Read the model definition and answer for the solid it produces. Units are mm, in the model's axes. A direction names the side the tool comes from. Give positions to 0.01 mm unless a question says otherwise; leave off trailing zeros. Write each loop counter-clockwise with the first axis right and the second up, starting at its lowest first coordinate (ties: lowest second). Pieces come first, ordered by that corner, then holes. Notation, with made-up numbers: M 13.25,79.5 L 61.25,79.5 A23 cw 61.25,94.5 Z; hole C 77.5,25 d3. An arc over 180 degrees is marked long. Put each result on its own line as item: value.
Autodesk Inventor part; units mm, degrees
ref_plane "YZ Plane" through (0, 0, 0) normal (1, 0, 0) x (0, 1, 0)
ref_plane "XZ Plane" through (0, 0, 0) normal (0, 1, 0) x (-1, 0, 0)
ref_plane "XY Plane" through (0, 0, 0) normal (0, 0, 1) x (1, 0, 0)
sketch "Sketch1" plane through (0, 0, 0) normal (0, 1, 0) x (-1, 0, 0)
  line L0 (0, 69.85) -> (0, -69.85)
  line L1 (2.54, 69.85) -> (10.16, 69.85)
  line L2 (10.16, 67.31) -> (10.16, 64.77)
  line L3 (10.16, 64.77) -> (7.9419, 64.217)
  line L4 (10.16, 58.674) -> (7.9419, 59.227)
  arc A0 (7.9419, 64.217) -> (7.9419, 59.227) centre (5.9783, 61.722) ccw
  line L5 (0, 69.85) -> (2.54, 69.85)
  line L6 (6.604, 69.85) -> (2.794, 69.85)
  line L7 (2.794, 69.85) -> (2.794, 82.55)
  line L8 (2.794, 82.55) -> (6.604, 82.55)
  line L9 (6.604, 82.55) -> (6.604, 69.85)
  line L10 (2.54, -69.85) -> (2.54, -81.28)
  line L11 (2.54, -81.28) -> (0, -81.28)
  line L12 (0, -81.28) -> (0, -69.85)
  line L13 (5.9783, 61.722) -> (7.9419, 61.722) construction
  line L14 (7.9419, 61.722) -> (7.9419, 59.227) construction
  line L15 (7.9419, 61.722) -> (7.9419, 64.217) construction
  line L16 (10.16, 67.31) -> (10.16, 69.85)
  line L17 (10.16, -66.802) -> (10.16, -69.85)
  line L18 (10.16, -69.85) -> (2.54, -69.85)
  line L19 (10.16, 58.674) -> (10.16, 56.134)
  line L20 (10.16, 56.134) -> (10.16, 53.594)
  line L21 (10.16, 53.594) -> (7.9419, 53.041)
  line L22 (7.9419, 50.546) -> (7.9419, 53.041) construction
  arc A1 (7.9419, 53.041) -> (7.9419, 48.051) centre (5.9783, 50.546) ccw
  line L23 (7.9419, 50.546) -> (7.9419, 48.051) construction
  line L24 (10.16, 47.498) -> (7.9419, 48.051)
  line L25 (10.16, 47.498) -> (10.16, 44.958)
  line L26 (5.9783, 50.546) -> (7.9419, 50.546) construction
  line L27 (10.16, 44.958) -> (10.16, 42.418)
  line L28 (10.16, 42.418) -> (7.9419, 41.865)
  line L29 (7.9419, 39.37) -> (7.9419, 41.865) construction
  arc A2 (7.9419, 41.865) -> (7.9419, 36.875) centre (5.9783, 39.37) ccw
  line L30 (7.9419, 39.37) -> (7.9419, 36.875) construction
  line L31 (10.16, 36.322) -> (7.9419, 36.875)
  line L32 (10.16, 36.322) -> (10.16, 33.782)
  line L33 (5.9783, 39.37) -> (7.9419, 39.37) construction
  line L34 (10.16, 33.782) -> (10.16, 31.242)
  line L35 (10.16, 31.242) -> (7.9419, 30.689)
  line L36 (7.9419, 28.194) -> (7.9419, 30.689) construction
  arc A3 (7.9419, 30.689) -> (7.9419, 25.699) centre (5.9783, 28.194) ccw
  line L37 (7.9419, 28.194) -> (7.9419, 25.699) construction
  line L38 (10.16, 25.146) -> (7.9419, 25.699)
  line L39 (10.16, 25.146) -> (10.16, 22.606)
  line L40 (5.9783, 28.194) -> (7.9419, 28.194) construction
  line L41 (10.16, 22.606) -> (10.16, 20.066)
  line L42 (10.16, 20.066) -> (7.9419, 19.513)
  line L43 (7.9419, 17.018) -> (7.9419, 19.513) construction
  arc A4 (7.9419, 19.513) -> (7.9419, 14.523) centre (5.9783, 17.018) ccw
  line L44 (7.9419, 17.018) -> (7.9419, 14.523) construction
  line L45 (10.16, 13.97) -> (7.9419, 14.523)
  line L46 (10.16, 13.97) -> (10.16, 11.43)
  line L47 (5.9783, 17.018) -> (7.9419, 17.018) construction
  line L48 (10.16, 11.43) -> (10.16, 8.89)
  line L49 (10.16, 8.89) -> (7.9419, 8.337)
  line L50 (7.9419, 5.842) -> (7.9419, 8.337) construction
  arc A5 (7.9419, 8.337) -> (7.9419, 3.347) centre (5.9783, 5.842) ccw
  line L51 (7.9419, 5.842) -> (7.9419, 3.347) construction
  line L52 (10.16, 2.794) -> (7.9419, 3.347)
  line L53 (10.16, 2.794) -> (10.16, 0.254)
  line L54 (5.9783, 5.842) -> (7.9419, 5.842) construction
  line L55 (10.16, 0.254) -> (10.16, -2.286)
  line L56 (10.16, -2.286) -> (7.9419, -2.839)
  line L57 (7.9419, -5.334) -> (7.9419, -2.839) construction
  arc A6 (7.9419, -2.839) -> (7.9419, -7.829) centre (5.9783, -5.334) ccw
  line L58 (7.9419, -5.334) -> (7.9419, -7.829) construction
  line L59 (10.16, -8.382) -> (7.9419, -7.829)
  line L60 (10.16, -8.382) -> (10.16, -10.922)
  line L61 (5.9783, -5.334) -> (7.9419, -5.334) construction
  line L62 (10.16, -10.922) -> (10.16, -13.462)
  line L63 (10.16, -13.462) -> (7.9419, -14.015)
  line L64 (7.9419, -16.51) -> (7.9419, -14.015) construction
  arc A7 (7.9419, -14.015) -> (7.9419, -19.005) centre (5.9783, -16.51) ccw
  line L65 (7.9419, -16.51) -> (7.9419, -19.005) construction
  line L66 (10.16, -19.558) -> (7.9419, -19.005)
  line L67 (10.16, -19.558) -> (10.16, -22.098)
  line L68 (5.9783, -16.51) -> (7.9419, -16.51) construction
  line L69 (10.16, -22.098) -> (10.16, -24.638)
  line L70 (10.16, -24.638) -> (7.9419, -25.191)
  line L71 (7.9419, -27.686) -> (7.9419, -25.191) construction
  arc A8 (7.9419, -25.191) -> (7.9419, -30.181) centre (5.9783, -27.686) ccw
  line L72 (7.9419, -27.686) -> (7.9419, -30.181) construction
  line L73 (10.16, -30.734) -> (7.9419, -30.181)
  line L74 (10.16, -30.734) -> (10.16, -33.274)
  line L75 (5.9783, -27.686) -> (7.9419, -27.686) construction
  line L76 (10.16, -33.274) -> (10.16, -35.814)
  line L77 (10.16, -35.814) -> (7.9419, -36.367)
  line L78 (7.9419, -38.862) -> (7.9419, -36.367) construction
  arc A9 (7.9419, -36.367) -> (7.9419, -41.357) centre (5.9783, -38.862) ccw
  line L79 (7.9419, -38.862) -> (7.9419, -41.357) construction
  line L80 (10.16, -41.91) -> (7.9419, -41.357)
  line L81 (10.16, -41.91) -> (10.16, -44.45)
  line L82 (5.9783, -38.862) -> (7.9419, -38.862) construction
  line L83 (10.16, -44.45) -> (10.16, -46.99)
  line L84 (10.16, -46.99) -> (7.9419, -47.543)
  line L85 (7.9419, -50.038) -> (7.9419, -47.543) construction
  arc A10 (7.9419, -47.543) -> (7.9419, -52.533) centre (5.9783, -50.038) ccw
  line L86 (7.9419, -50.038) -> (7.9419, -52.533) construction
  line L87 (10.16, -53.086) -> (7.9419, -52.533)
  line L88 (10.16, -53.086) -> (10.16, -55.626)
  line L89 (5.9783, -50.038) -> (7.9419, -50.038) construction
  line L90 (10.16, -55.626) -> (10.16, -58.166)
  line L91 (10.16, -58.166) -> (7.9419, -58.719)
  line L92 (7.9419, -61.214) -> (7.9419, -58.719) construction
  arc A11 (7.9419, -58.719) -> (7.9419, -63.709) centre (5.9783, -61.214) ccw
  line L93 (7.9419, -61.214) -> (7.9419, -63.709) construction
  line L94 (10.16, -64.262) -> (7.9419, -63.709)
  line L95 (10.16, -64.262) -> (10.16, -66.802)
  line L96 (5.9783, -61.214) -> (7.9419, -61.214) construction
  point P0 (0, 0)
  point P1 (2.794, 69.85)
  dimension "d1" = 7.62
  dimension "d5" = 104
  dimension "d7" = 3.175
  dimension "d8" = 2.286
  dimension "d12" = 2.54
  dimension "d27" = 12.7
  dimension "d28" = 3.81
  dimension "d29" = 2.794
  dimension "d66" = 139.7
  dimension "d67" = 69.85
  dimension "d76" = 10.16
  dimension "d77" = 2.54
  dimension "d87" = 11.43
  dimension "d88" = 2.54
  dimension "d89" = 4.9899
  dimension "d90" = 2.54
  dimension "d91" = 11.176
  dimension "d94" = 11.176
extrude "Extrusion1" add sketch "Sketch1" along normal blind 11.1125
sketch "Sketch3" plane through (0, 0, 69.85) normal (1, 0, 0) x (0, 0, -1)
  line L0 (158.877, 5.5563) -> (143.383, 5.5562) construction
  line L1 (158.877, 8.9853) -> (143.383, 8.9852)
  line L2 (143.383, 2.1272) -> (158.877, 2.1273)
  arc A0 (158.877, 2.1273) -> (158.877, 8.9853) centre (158.877, 5.5563) ccw
  arc A1 (143.383, 8.9852) -> (143.383, 2.1272) centre (143.383, 5.5562) ccw
  line L3 (151.13, 0) -> (151.13, 11.1125)
  line L4 (0, 11.1125) -> (151.13, 11.1125)
  line L5 (-20.447, 5.5563) -> (-4.953, 5.5563) construction
  line L6 (-20.447, 2.1273) -> (-4.953, 2.1272)
  line L7 (-4.953, 8.9853) -> (-20.447, 8.9853)
  arc A2 (-20.447, 8.9853) -> (-20.447, 2.1273) centre (-20.447, 5.5563) ccw
  arc A3 (-4.953, 2.1272) -> (-4.953, 8.9853) centre (-4.953, 5.5563) ccw
  line L8 (-12.7, 0) -> (-12.7, 11.1125)
  point P0 (69.85, 0)
  point P1 (151.13, 5.5563)
  point P2 (-12.7, 5.5563)
  point P3 (-12.7, 8.9853)
  point P4 (-12.7, 2.1272)
  point P5 (151.13, 2.1272)
  point P6 (151.13, 8.9853)
  dimension "d45" = 11.1125
  dimension "d46" = 5.5563
  dimension "d47" = 7.747
  dimension "d48" = 7.747
  dimension "d49" = 6.858
  dimension "d50" = 6.858
extrude "Extrusion2" cut sketch "Sketch3" against normal through all contours L3 L2 A1 L1 | L8 L7 A3 L6
properties part number "Hose Clamp V4" material "ABS Plastic"
(1) Section A-A on z = 39.37 is taken. Determine the outline of the cut face in (x, y), and give its area (3 significant figures).
Result:
outline: M -2.8,0 L 0,0 L 0,11.11 L -2.8,11.11 Z
area: 31.2 mm²
(2) Section B-B on x = -4.75 is taken. Give the number of separate pieces and of enclosed holes in the cut face, and give its area (3 significant figures).
Result:
separate pieces: 13
enclosed holes: 0
area: 841 mm²
(3) Which of the six approach directions +Z, -Z, +X, -X, +Y, -Y give full straight-line access (tool end or side, diameter ignored) to faces 5 (the face through (-2.54, 1.8, -75.5)), 6 (the face through (-5, 8.985, 79)), 7 (the face through (-6.604, 1.8, 74.9)), 8 (the face through (-2.794, 1.8, 74.7))?
Result:
face 5: -Z, -X, +Y, -Y
face 6: +Z, +X, -X
face 7: +Z, -X, +Y, -Y
face 8: +Z, +X, +Y, -Y
(4) For a pull along X with two mould halves and no side action, classify faces 1 (the face through (-10.16, 5, 0)), 2 (the face through (-6, 5, -69.85)), 3 (the face through (-2.805, 5.478, -5.433)), 4 (the face through (-2.805, 5.478, -38.961)) as +X half, -X half, draft (parallel to the pull), parting line (faces both ways), or undercut.
Result:
face 1: -X half
face 2: draft
face 3: undercut
face 4: undercut
(5) Straight lines are drawn through the part: line 1 along Y through (x, z) = (-1.5, -71.5); line 2 along Z through (x, y) = (-2.5, 1); line 3 along X through (y, z) = (6.5, 28.5). For each, find the intervals that lie inside material, in ascending order. Write a range as from..to.
Result:
line 1: y = 0..2.79, 8.32..11.11
line 2: z = -81.28..69.85
line 3: x = -2.82..0
(6) Section C-C on z = -51 is taken. Determine the outline of the cut face in (x, y).
Result:
outline: M -2.95,0 L 0,0 L 0,11.11 L -2.95,11.11 Z
(7) Given pin 1 Ø5.5 at (y, z) = (7, 74.5) entering from +X; pin 2 Ø2 at (x, y) = (-2.5, 4.5) entering from +Z; pin 3 Ø5 at (y, z) = (7.5, -63) entering from +X; pin 4 Ø3.5 at (y, z) = (7.5, 76) entering from -X, each flat-ended and moving along its own axis, determine where each tip first touches the part or whether it passes through.
Result:
pin 1: stops at x = -2.79
pin 2: stops at z = 72.03
pin 3: stops at x = 0
pin 4: stops at x = -6.6
